Study the drawing (mm; zero at the part's minimum x, y, z) and answer. A direction names the side the tool comes from. Coordinates: 2 decimals unless noted, no trailing zeros. Order: outer loops, then holes, each group sorted by start corner. A loop starts at its lowest first (then second) coordinate and runs counter-clockwise, first axis right, second up. Notation, with made-up numbers: M -24,12 L -18,12 A10 ccw -18,27 Z; hole C -22.5,37.25 d1. An arc over 180 degrees is marked long. One line per item, written item: value. Start each with the question number.
Q1. The part is cut by section B-B on z = 28. Give the vertices of the cut face in (x, y).
Q2. Straight lines are drawn through the part: line 1 along Y through (x, z) = (14.25, 28); line 2 along X through (y, z) = (1, 8); line 3 along X through (y, z) = (9.5, 2.5). For each, find the intervals that lie inside material, in ascending order. Write a range as [from, to].
Q3. The part is cut by section C-C on z = 8. Give the vertices of the cut face in (x, y).
Q4. The part is cut by section A-A on y = 39. Give the vertices of the cut face in (x, z).
Q5. The part is cut by section D-D on y = 27.5. Give the vertices of the cut face in (x, z).
Q6. Each of these flat-tipped pins is pushed along its axis until it touches: pin 1 Ø5 at (y, z) = (27.5, 13.5) entering from -X; pin 2 Ø2.5 at (x, z) = (7.5, 18) entering from +Y; pin 3 Ø8 at (x, z) = (11, 8) entering from -Y; pin 4 Ø0.6 at (x, z) = (14, 29) entering from -Y. Where does it stop, or does it pass through?
Q7. For the marked faces 1 and 2, determine the directions among +Z, -Z, +X, -X, +Y, -Y from which every point of the face is accessible in a straight line to the end or side of a thin tool.
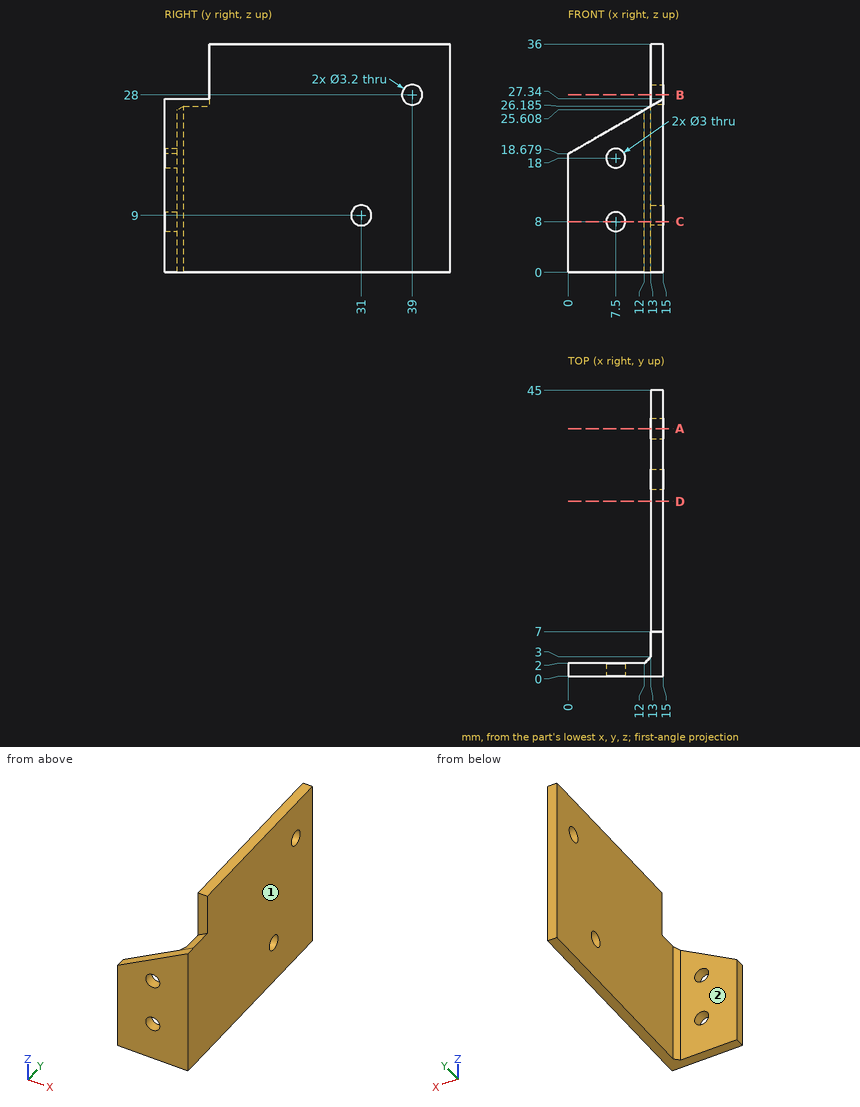
Output:
1. outline: M 13,7 L 15,7 L 15,37.4 L 13,37.4 Z; M 13,40.6 L 15,40.6 L 15,45 L 13,45 Z
2. line 1: y = [7, 37.4], [40.6, 45]
2. line 2: x = [0, 6], [9, 15]
2. line 3: x = [13, 15]
3. outline: M 0,0 L 6,0 L 6,2 L 0,2 Z; M 9,0 L 15,0 L 15,29.75 L 13,29.75 L 13,3 L 12,2 L 9,2 Z; M 13,32.25 L 15,32.25 L 15,45 L 13,45 Z
4. outline: M 13,0 L 15,0 L 15,26.4 L 13,26.4 Z; M 13,29.6 L 15,29.6 L 15,36 L 13,36 Z
5. outline: M 13,0 L 15,0 L 15,36 L 13,36 Z
6. pin 1: stops at x = 13
6. pin 2: passes through
6. pin 3: stops at y = 0
6. pin 4: stops at y = 7
7. face 1: +Z, -Z, +X, +Y, -Y
7. face 2: +Z, -Z, -X, +Y
